from build123d import *

# Parameters (mm, degrees)
SKETCH1_W           = 40
SKETCH1_H           = 40
BOSS_EXTRUDE1_DEPTH = 15
SKETCH3_R           = 2.75
BOSS_EXTRUDE2_DEPTH = 5
FILLET1_R           = 1
SKETCH4_R           = 12.5
CUT_EXTRUDE1_DEPTH  = 3.5
SKETCH5_R           = 8.5
CUT_EXTRUDE2_DEPTH  = 41
SKETCH6_R           = 3
CUT_EXTRUDE3_DEPTH  = 2
SKETCH7_R           = 1.75
CUT_EXTRUDE4_DEPTH  = 16


with BuildPart() as part:
    # Sketch1 → Boss-Extrude1 (new body)
    with BuildSketch(Plane.XY):
        Rectangle(SKETCH1_W, SKETCH1_H)
    extrude(amount=BOSS_EXTRUDE1_DEPTH)

    # Sketch3 → Boss-Extrude2 (add)
    with BuildSketch(Plane(origin=(0, 0, 0), x_dir=(-1, 0, 0), z_dir=(0, 0, -1))):
        with Locations(Location((-15, 15, 0), (0, 0, 180))):  # turned: the seam where the file's is
            Circle(SKETCH3_R)
        with Locations(Location((15, 15, 0), (0, 0, 180))):  # turned: the seam where the file's is
            Circle(SKETCH3_R)
        with Locations(Location((-15, -15, 0), (0, 0, 180))):  # turned: the seam where the file's is
            Circle(SKETCH3_R)
        with Locations(Location((15, -15, 0), (0, 0, 180))):  # turned: the seam where the file's is
            Circle(SKETCH3_R)
    extrude(amount=BOSS_EXTRUDE2_DEPTH)

    # Fillet1
    fillet1_edges = [part.edges().sort_by_distance(p)[0] for p in [
        (12.25, 15, -5),
        (-17.75, 15, -5),
        (12.25, -15, -5),
        (-17.75, -15, -5),
    ]]
    fillet(fillet1_edges, radius=FILLET1_R)

    # Sketch4 → Cut-Extrude1 (cut)
    with BuildSketch(Plane(origin=(0, 0, 0), x_dir=(-1, 0, 0), z_dir=(0, 0, -1))):
        Circle(SKETCH4_R)
    extrude(amount=-CUT_EXTRUDE1_DEPTH, mode=Mode.SUBTRACT)

    # Sketch5 → Cut-Extrude2 (cut, through all)
    with BuildSketch(Plane(origin=(0, 20, 0), x_dir=(1, 0, 0), z_dir=(0, 1, 0))):
        with Locations((0, -18)):
            Circle(SKETCH5_R)
    extrude(amount=-CUT_EXTRUDE2_DEPTH, mode=Mode.SUBTRACT)

    # Sketch6 → Cut-Extrude3 (cut)
    with BuildSketch(Plane(origin=(0, 0, 0), x_dir=(-1, 0, 0), z_dir=(0, 0, -1))):
        with Locations((-16.5, 0)):
            Circle(SKETCH6_R)
        with Locations((16.5, 0)):
            Circle(SKETCH6_R)
    extrude(amount=-CUT_EXTRUDE3_DEPTH, mode=Mode.SUBTRACT)

    # Sketch7 → Cut-Extrude4 (cut, through all)
    with BuildSketch(Plane(origin=(0, 0, 0), x_dir=(-1, 0, 0), z_dir=(0, 0, -1))):
        with Locations((16.5, 0)):
            Circle(SKETCH7_R)
        with Locations((-16.5, 0)):
            Circle(SKETCH7_R)
    extrude(amount=-CUT_EXTRUDE4_DEPTH, mode=Mode.SUBTRACT)


solid = part.part
Work out the finished part from the listing and answer in its coordinate system (mm). A direction names the side the tool comes from. Give positions to 0.01 mm unless a question says otherwise; leave off trailing zeros. Write each loop counter-clockwise with the first axis right and the second up, starting at its lowest first coordinate (ties: lowest second). Pieces come first, ordered by that corner, then holes. Notation, with made-up numbers: M 15.5,46 L 24.5,46 A16 cw 24.5,74 Z; hole C 9.25,70 d6. An arc over 180 degrees is marked long. Answer as CSV lines item,"result".
Q1. A cutting plane is placed at B-B on y = 0. Write down the section's boundary in (x, z).
A:
outline,"M -20,0 L -19.5,0 L -19.5,2 L -18.25,2 L -18.25,15 L -20,15 Z; M -14.75,2 L -13.5,2 L -13.5,0 L -12.5,0 L -12.5,3.5 L 12.5,3.5 L 12.5,0 L 13.5,0 L 13.5,2 L 14.75,2 L 14.75,15 L 7.95,15 A8.5 cw -7.95,15 L -14.75,15 Z; M 18.25,2 L 19.5,2 L 19.5,0 L 20,0 L 20,15 L 18.25,15 Z"
Q2. The mould has two halves that part along Y. Classify faces 3 (the flat face through (0, -20, 7)), 4 (the cylindrical face through (0.1, 0.3, 9.5)), 5 (the cylindrical face through (12.973, -16.859, -1.972)): +Y half, -Y half, draft (parallel to the pull), parting line (faces both ways), or undercut.
A:
face 3,"-Y half"
face 4,"draft"
face 5,"undercut"
Q3. A cutting plane is placed at A-A on z = 11.75. Write down the section's boundary in (x, y), plus the area to 3 significant figures.
A:
outline,"M -20,-20 L -5.76,-20 L -5.76,20 L -20,20 Z; M 5.76,-20 L 20,-20 L 20,20 L 5.76,20 Z; hole C -16.5,0 d3.5; hole C 16.5,0 d3.5"
area,"1,120 mm²"
Q4. A cutting plane is placed at D-D on x = 0. Write down the section's boundary in (y, z).
A:
outline,"M -20,0 L -12.5,0 L -12.5,3.5 L 12.5,3.5 L 12.5,0 L 20,0 L 20,9.5 L -20,9.5 Z"
Q5. Find the intervals of material crossed by probe 1 along Y at (x, z) = (0, 2.75); probe 2 along Y at (x, z) = (16.5, 1.3); probe 3 along Z at (x, y) = (9.5, -2.5), in increasing order. Write a range as [from, to].
A:
probe 1,"y = [-20, -12.5], [12.5, 20]"
probe 2,"y = [-20, -3], [3, 20]"
probe 3,"z = [3.5, 15]"
Q6. A tool of negligible diameter and unlimited length cuts with its end or side. For faces 1 (the cylindrical face through (-11.923, 3.755, 1.726)), 2 (the flat face through (-15, 15, -5)), from which of +Z, -Z, +X, -X, +Y, -Y can it reach the whole face along a straight path? Write none if from no direction.
A:
face 1,"-Z"
face 2,"-Z, +X, -X, +Y, -Y"
Q7. A cutting plane is placed at C-C on z = 1.5. Write down the section's boundary in (x, y), plus the area to 3 significant figures.
A:
outline,"M -20,-20 L 20,-20 L 20,20 L -20,20 Z; hole C -16.5,0 d6; hole C 0,0 d25; hole C 16.5,0 d6"
area,"1,050 mm²"
Q8. Given P1, Ø20, axis at x = 0, y = 0, coming from the -Z side; P2, Ø1, axis at x = 15.5, z = -1, coming from the -Y side; P3, Ø7, axis at x = -16.5, y = 0, coming from the -Z side; P4, Ø3, axis at x = -16.5, y = 0, coming from the -Z side, each flat-ended and moving along its own axis, determine where each tip first touches the part or whether it passes through.
A:
P1,"stops at z = 3.5"
P2,"stops at y = -17.75"
P3,"stops at z = 0"
P4,"passes through"
